Source: CAD feature listing. Evaluate the final solid. Frame: model axes, mm. A direction names the side the tool comes from. Give positions to 0.01 mm unless a question says otherwise; leave off trailing zeros. Loops run counter-clockwise (first coordinate to the right, second up) from the corner with the lowest first, then second, coordinate; pieces in that order, holes last. Notation, with made-up numbers: (-24, -6.75) -> (-18, -6.75) arc R31 ccw to (-18, 27.25) -> close; hole circle Ø7 at (-0.75, 53.5). An arc over 180 degrees is marked (long way). Return JSON: item names as keys, results as strings. Group by question number.
(1) Cut plane D-D on x = -35.5. Return loops of the section in (y, z), then the cut area to 3 significant figures.
(2) Cut plane A-A on y = -0.9. Return loops of the section in (x, z).
(3) Pin query (flat end, axial travel): pin 1 (0.6 mm diameter, centred on x = -29.5, y = -1.5, fed in from +Z); pin 2 (1 mm diameter, centred on x = -34, y = -1, fed in from -Z). Return the tip coordinate at first contact, or that it passes through.
(4) Cut plane B-B on z = 25. Return loops of the section in (x, y).
(5) Cut plane C-C on x = -18. Return loops of the section in (y, z).
(6) Access query for faces 1 (the face through (-36, -1, 25.746)), 2 (the face through (-36, -2, 30)), 3 (the face through (-36, -1, 34.746)). Directions: +Z, -Z, +X, -X, +Y, -Y. A direction counts if a zero-diameter tool reaches every point of the face in a straight line with its end or side. Return the directions, or none.
(7) Draft query along X for faces 4 (the face through (-36, 0, 30)), 5 (the face through (-17.69, -0.99, 29.27)). Return one class per face: released by +X, released by -X, zero draft, split by the parting line, or undercut.
(8) Ray query, line 1 (Z direction, x = -18, y = -1.3); line 2 (X direction, y = -0.15, z = 30); line 3 (Z direction, x = -47, y = -1.7). Return the intervals inside material, ascending. Write a range as from..to.
```python
from build123d import *

# Parameters (mm, degrees)
F0_R     = 1
F1_DEPTH = 2


with BuildPart() as f1:
    # F0 (on Front) → F1 (new body)
    with BuildSketch(Plane.XZ):
        with BuildLine():
            ThreePointArc((-49.9391267766, 34.7456367077), (-53.9077537432, 36.2456367077), (-57.8763807098, 34.7456367077))
            Line((-57.8763807098, 34.7456367077), (-49.9391267766, 34.7456367077))
        make_face()
        with BuildLine():
            Line((-49.9391267766, 34.7456367077), (-57.8763807098, 34.7456367077))
            ThreePointArc((-57.8763807098, 34.7456367077), (-58.4309342214, 34.1878237101), (-58.9077537432, 33.562261498))
            Line((-58.9077537432, 33.562261498), (-58.9077537432, 26.9290119173))
            ThreePointArc((-58.9077537432, 26.9290119173), (-58.4309342214, 26.3034497053), (-57.8763807098, 25.7456367077))
            Line((-57.8763807098, 25.7456367077), (-49.9391267766, 25.7456367077))
            ThreePointArc((-49.9391267766, 25.7456367077), (-49.3845732651, 26.3034497053), (-48.9077537432, 26.9290119173))
            Line((-48.9077537432, 26.9290119173), (-48.9077537432, 30.2456367077))
            Line((-48.9077537432, 30.2456367077), (-48.9077537432, 33.562261498))
            ThreePointArc((-48.9077537432, 33.562261498), (-49.3845732651, 34.1878237101), (-49.9391267766, 34.7456367077))
        make_face()
        with Locations((-53.9077537432, 30.2456367077)):
            Circle(F0_R, mode=Mode.SUBTRACT)
        with BuildLine():
            Line((-58.9077537432, 26.9290119173), (-58.9077537432, 33.562261498))
            ThreePointArc((-58.9077537432, 33.562261498), (-59.9077537432, 30.2456367077), (-58.9077537432, 26.9290119173))
        make_face()
        with BuildLine():
            Line((-48.9077537432, 34.7456367077), (-49.9391267766, 34.7456367077))
            ThreePointArc((-49.9391267766, 34.7456367077), (-49.3845732651, 34.1878237101), (-48.9077537432, 33.562261498))
            Line((-48.9077537432, 33.562261498), (-48.9077537432, 34.7456367077))
        make_face()
        with BuildLine():
            Line((-22.9077537432, 34.7456367077), (-48.9077537432, 34.7456367077))
            Line((-48.9077537432, 34.7456367077), (-48.9077537432, 33.562261498))
            ThreePointArc((-48.9077537432, 33.562261498), (-48.1631910967, 31.9776875152), (-47.9077537432, 30.2456367077))
            ThreePointArc((-47.9077537432, 30.2456367077), (-48.1631910967, 28.5135859001), (-48.9077537432, 26.9290119173))
            Line((-48.9077537432, 26.9290119173), (-48.9077537432, 25.7456367077))
            Line((-48.9077537432, 25.7456367077), (-22.9077537432, 25.7456367077))
            Line((-22.9077537432, 25.7456367077), (-22.9077537432, 26.9290119173))
            ThreePointArc((-22.9077537432, 26.9290119173), (-23.9077537432, 30.2456367077), (-22.9077537432, 33.562261498))
            Line((-22.9077537432, 33.562261498), (-22.9077537432, 34.7456367077))
        make_face()
        with BuildLine():
            ThreePointArc((-47.9077537432, 30.2456367077), (-48.1631910967, 31.9776875152), (-48.9077537432, 33.562261498))
            Line((-48.9077537432, 33.562261498), (-48.9077537432, 30.2456367077))
            Line((-48.9077537432, 30.2456367077), (-48.9077537432, 26.9290119173))
            ThreePointArc((-48.9077537432, 26.9290119173), (-48.1631910967, 28.5135859001), (-47.9077537432, 30.2456367077))
        make_face()
        with BuildLine():
            Line((-49.9391267766, 25.7456367077), (-57.8763807098, 25.7456367077))
            ThreePointArc((-57.8763807098, 25.7456367077), (-53.9077537432, 24.2456367077), (-49.9391267766, 25.7456367077))
        make_face()
        with BuildLine():
            Line((-21.8763807098, 34.7456367077), (-22.9077537432, 34.7456367077))
            Line((-22.9077537432, 34.7456367077), (-22.9077537432, 33.562261498))
            ThreePointArc((-22.9077537432, 33.562261498), (-22.4309342214, 34.1878237101), (-21.8763807098, 34.7456367077))
        make_face()
        with BuildLine():
            ThreePointArc((-48.9077537432, 26.9290119173), (-49.3845732651, 26.3034497053), (-49.9391267766, 25.7456367077))
            Line((-49.9391267766, 25.7456367077), (-48.9077537432, 25.7456367077))
            Line((-48.9077537432, 25.7456367077), (-48.9077537432, 26.9290119173))
        make_face()
        with BuildLine():
            ThreePointArc((-13.9391267766, 34.7456367077), (-17.9077537432, 36.2456367077), (-21.8763807098, 34.7456367077))
            Line((-21.8763807098, 34.7456367077), (-13.9391267766, 34.7456367077))
        make_face()
        with BuildLine():
            Line((-13.9391267766, 34.7456367077), (-21.8763807098, 34.7456367077))
            ThreePointArc((-21.8763807098, 34.7456367077), (-22.4309342214, 34.1878237101), (-22.9077537432, 33.562261498))
            Line((-22.9077537432, 33.562261498), (-22.9077537432, 30.2456367077))
            Line((-22.9077537432, 30.2456367077), (-22.9077537432, 26.9290119173))
            ThreePointArc((-22.9077537432, 26.9290119173), (-22.4309342214, 26.3034497053), (-21.8763807098, 25.7456367077))
            Line((-21.8763807098, 25.7456367077), (-13.9391267766, 25.7456367077))
            ThreePointArc((-13.9391267766, 25.7456367077), (-13.3845732651, 26.3034497053), (-12.9077537432, 26.9290119173))
            Line((-12.9077537432, 26.9290119173), (-12.9077537432, 33.562261498))
            ThreePointArc((-12.9077537432, 33.562261498), (-13.3845732651, 34.1878237101), (-13.9391267766, 34.7456367077))
        make_face()
        with BuildLine():
            ThreePointArc((-16.9077537432, 30.2456367077), (-17.9077537432, 29.2456367077), (-18.9077537432, 30.2456367077))
            ThreePointArc((-18.9077537432, 30.2456367077), (-17.9077537432, 31.2456367077), (-16.9077537432, 30.2456367077))
        make_face(mode=Mode.SUBTRACT)
        with BuildLine():
            Line((-22.9077537432, 30.2456367077), (-22.9077537432, 33.562261498))
            ThreePointArc((-22.9077537432, 33.562261498), (-23.9077537432, 30.2456367077), (-22.9077537432, 26.9290119173))
            Line((-22.9077537432, 26.9290119173), (-22.9077537432, 30.2456367077))
        make_face()
        with BuildLine():
            ThreePointArc((-21.8763807098, 25.7456367077), (-22.4309342214, 26.3034497053), (-22.9077537432, 26.9290119173))
            Line((-22.9077537432, 26.9290119173), (-22.9077537432, 25.7456367077))
            Line((-22.9077537432, 25.7456367077), (-21.8763807098, 25.7456367077))
        make_face()
        with BuildLine():
            ThreePointArc((-11.9077537432, 30.2456367077), (-12.1631910967, 31.9776875152), (-12.9077537432, 33.562261498))
            Line((-12.9077537432, 33.562261498), (-12.9077537432, 26.9290119173))
            ThreePointArc((-12.9077537432, 26.9290119173), (-12.1631910967, 28.5135859001), (-11.9077537432, 30.2456367077))
        make_face()
        with BuildLine():
            Line((-13.9391267766, 25.7456367077), (-21.8763807098, 25.7456367077))
            ThreePointArc((-21.8763807098, 25.7456367077), (-17.9077537432, 24.2456367077), (-13.9391267766, 25.7456367077))
        make_face()
    extrude(amount=F1_DEPTH)


solid = f1.part
```
Answers:
{
 "1": {"outline": "(-2, 25.75) -> (0, 25.75) -> (0, 34.75) -> (-2, 34.75) -> close", "area": "18.0 mm²"},
 "2": {"outline": "(-49.94, 25.75) -> (-21.88, 25.75) arc R6 ccw (long way) to (-21.88, 34.75) -> (-49.94, 34.75) arc R6 ccw (long way) to start; hole circle Ø2 at (-53.91, 30.25); hole circle Ø2 at (-17.91, 30.25)"},
 "3": {"pin 1": "z = 34.75", "pin 2": "z = 25.75"},
 "4": {"outline": "(-56.82, -2) -> (-51, -2) -> (-51, 0) -> (-56.82, 0) -> close; (-20.82, -2) -> (-15, -2) -> (-15, 0) -> (-20.82, 0) -> close"},
 "5": {"outline": "(-2, 24.25) -> (0, 24.25) -> (0, 29.25) -> (-2, 29.25) -> close; (-2, 31.24) -> (0, 31.24) -> (0, 36.24) -> (-2, 36.24) -> close"},
 "6": {"face 1": "-Z, +Y, -Y", "face 2": "+Z, -Z, +X, -X, -Y", "face 3": "+Z, +Y, -Y"},
 "7": {"face 4": "zero draft", "face 5": "undercut"},
 "8": {"line 1": "24.25..29.25, 31.24..36.24", "line 2": "-59.9..-54.88, -52.94..-18.88, -16.94..-11.91", "line 3": "25.75..34.75"}
}
